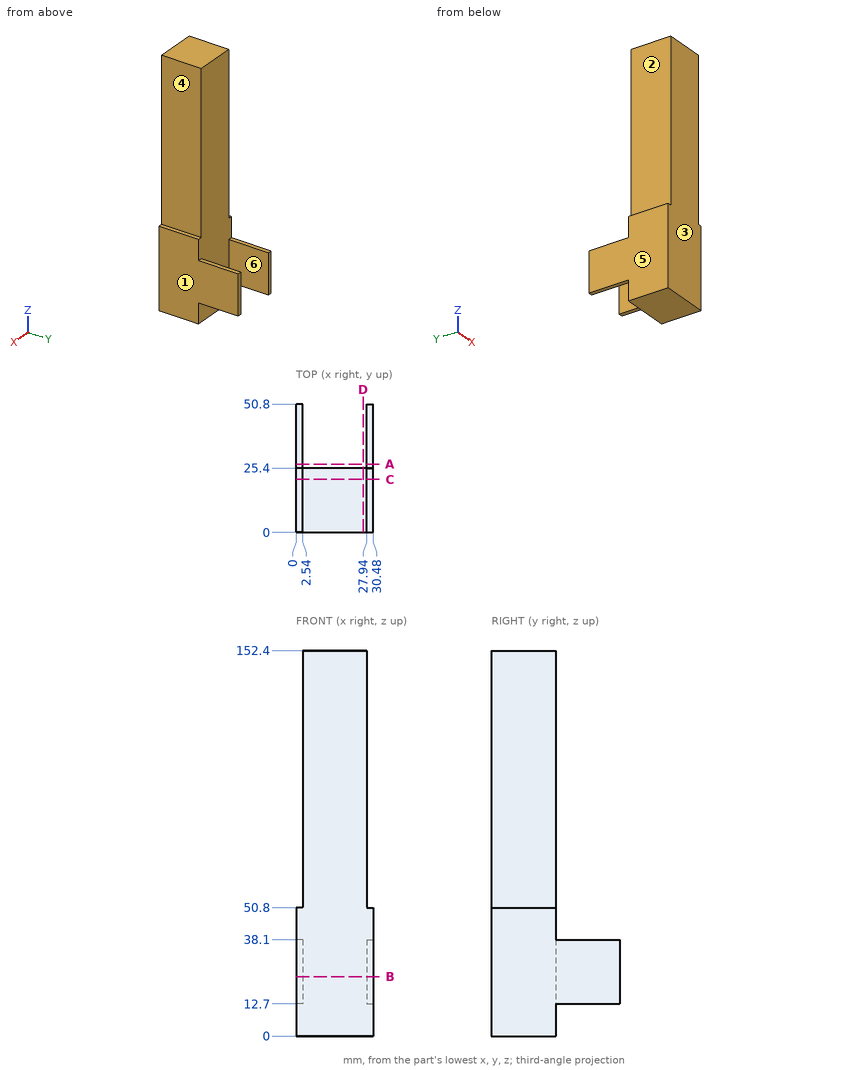
Input: dimensioned drawing with shaded views. Units: mm. Origin: part minimum x, y, z. A direction names the side the tool comes from. Give positions to 0.01 mm unless a question says otherwise; leave off trailing zeros. Order: outer loops, then holes, each group sorted by start corner. A loop starts at its lowest first (then second) coordinate and runs counter-clockwise, first axis right, second up. Notation, with made-up numbers: (16, -6) -> (32, -6) arc R30 ccw to (32, 19) -> close; hole circle Ø11 at (69, 78). An arc over 180 degrees is marked (long way). Write item = value, one per line.
Item 1: Section query B-B (z = 23.5). Output: boundary loops of the cut face in (x, y).
Check result:
outline = (0, 0) -> (30.48, 0) -> (30.48, 50.8) -> (27.94, 50.8) -> (27.94, 25.4) -> (2.54, 25.4) -> (2.54, 50.8) -> (0, 50.8) -> close
Item 2: Mould query, pull axis X, two halves, no side actions, for the marked faces 3, 4, 5 and 6. Classes: +X half, -X half, draft (parallel to the pull), parting line (faces both ways), or undercut.
Check result:
face_3 = draft
face_4 = +X half
face_5 = -X half
face_6 = undercut
Item 3: Ray query, probe 1 along X at (y, z) = (15, 85); probe 2 along X at (y, z) = (41, 37); probe 3 along Y at (x, z) = (24.5, 78). Return the intervals inside material, ascending.
Check result:
probe_1 = 2.54 to 27.94
probe_2 = 0 to 2.54, 27.94 to 30.48
probe_3 = 0 to 25.4
Item 4: Section query C-C (y = 21). Output: boundary loops of the cut face in (x, z).
Check result:
outline = (0, 0) -> (30.48, 0) -> (30.48, 50.8) -> (27.94, 50.8) -> (27.94, 152.4) -> (2.54, 152.4) -> (2.54, 50.8) -> (0, 50.8) -> close
Item 5: Section query A-A (y = 27). Output: boundary loops of the cut face in (x, z).
Check result:
outline = (0, 12.7) -> (2.54, 12.7) -> (2.54, 38.1) -> (0, 38.1) -> close; (27.94, 12.7) -> (30.48, 12.7) -> (30.48, 38.1) -> (27.94, 38.1) -> close
Item 6: Section query D-D (x = 26.5). Output: boundary loops of the cut face in (y, z).
Check result:
outline = (0, 0) -> (25.4, 0) -> (25.4, 152.4) -> (0, 152.4) -> close
Item 7: Set-up query: the marked faces 1 and 2. Return all of +Z, -Z, +X, -X, +Y, -Y with unobstructed straight access to the full face (end or side cutting, diameter ignored); none if empty.
Check result:
face_1 = +Z, -Z, +X, +Y, -Y
face_2 = +Z, -X, +Y, -Y
Item 8: Contact query for flat-ended pins moving along their axis: pin 1 (1.3 mm diameter, centred on x = 0.5, y = 41, fed in from +Z); pin 2 (2 mm diameter, centred on x = 7, z = 40, fed in from +Y); pin 3 (2 mm diameter, centred on y = 11, z = 114, fed in from +X). Output: stop coordinate, or through.
Check result:
pin_1 = 38.1
pin_2 = 25.4
pin_3 = 27.94
